```python
from build123d import *

# Parameters (mm, degrees)
SKETCH1_R          = 2.5
BASE_FLANGE1_DEPTH = 3


# Sheet-metal steps are written as plain solids
with BuildPart() as part:
    # Sketch1 → Base-Flange1 (new body)
    with BuildSketch(Plane(origin=(0, 0, 0), x_dir=(1, 0, 0), z_dir=(0, 1, 0))):
        with BuildLine():
            Line((-50, 10), (50, 10))
            ThreePointArc((50, 10), (60, 0), (50, -10))
            Line((50, -10), (-50, -10))
            ThreePointArc((-50, -10), (-60, 0), (-50, 10))
        make_face()
        with Locations(Location((-50, 0, 0), (0, 0, 270))):
            Circle(SKETCH1_R, mode=Mode.SUBTRACT)
        with BuildLine():
            Line((-25, 2.5), (45, 2.5))
            ThreePointArc((45, 2.5), (47.5, 0), (45, -2.5))
            Line((45, -2.5), (-25, -2.5))
            ThreePointArc((-25, -2.5), (-27.5, 0), (-25, 2.5))
        make_face(mode=Mode.SUBTRACT)
    extrude(amount=-BASE_FLANGE1_DEPTH)


solid = part.part
```
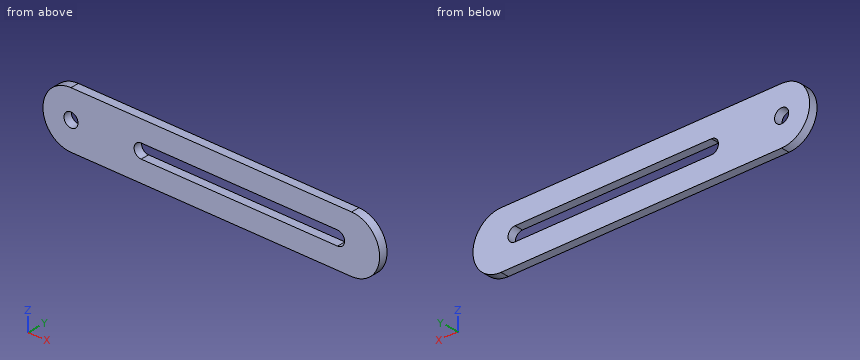
Could you check a few things on this model? Use its own coordinates, in mm. Round coordinates to 2 decimals unless told otherwise and drop trailing zeros. Loops run counter-clockwise (first coordinate to the right, second up) from the corner with the lowest first, then second, coordinate; pieces in that order, holes last.
Q1. Please list where these lines run through material, in increasing order: L1, parallel to X at y = -0.65, z = 0; L2, parallel to Z at x = 33.5, y = -0.8; L3, parallel to X at y = -2.5, z = -1.
Q2. I want a section at B-B (y = -1.5). Write out the boundary of the cut face in (x, z), and give its area (3 significant figures).
Q3. I want a section at D-D (z = -6.25). Write out the boundary of the cut face in (x, y).
Q4. I want a section at C-C (z = 0.25). Write out the boundary of the cut face in (x, y), and give its area (3 significant figures).
Q5. I want a section at A-A (x = 5). Write out the boundary of the cut face in (y, z), and give its area (3 significant figures).
Answer below:
1. L1: x = -60 to -52.5, -47.5 to -27.5, 47.5 to 60
1. L2: z = -10 to -2.5, 2.5 to 10
1. L3: x = -59.95 to -52.29, -47.71 to -27.29, 47.29 to 59.95
2. outline: (-50, -10) - (50, -10) arc R10 ccw to (50, 10) - (-50, 10) arc R10 ccw to start; hole circle Ø5 at (-50, 0); hole (-25, -2.5) - (45, -2.5) arc R2.5 ccw to (45, 2.5) - (-25, 2.5) arc R2.5 ccw to start
2. area: 1,920 mm2
3. outline: (-57.81, -3) - (57.81, -3) - (57.81, 0) - (-57.81, 0) - close
4. outline: (-60, -3) - (-52.49, -3) - (-52.49, 0) - (-60, 0) - close; (-47.51, -3) - (-27.49, -3) - (-27.49, 0) - (-47.51, 0) - close; (47.49, -3) - (60, -3) - (60, 0) - (47.49, 0) - close
4. area: 120 mm2
5. outline: (-3, -10) - (0, -10) - (0, -2.5) - (-3, -2.5) - close; (-3, 2.5) - (0, 2.5) - (0, 10) - (-3, 10) - close
5. area: 45.0 mm2
